Source: CAD feature listing. Evaluate the final solid. Frame: model axes, mm. Round coordinates to 2 decimals unless told otherwise and drop trailing zeros. Loops run counter-clockwise (first coordinate to the right, second up) from the corner with the lowest first, then second, coordinate; pieces in that order, holes last. Notation, with made-up numbers: M -13.75,12.25 L 11.25,12.25 A18 cw 11.25,25.25 Z; hole C -3,63 d3. An arc over 180 degrees is marked long. Write each question's results on one line, items separated by ' | '. Start each with the question number.
1. Section B-B on x = -120. Output: boundary loops of the cut face in (y, z) (1 decimal).
2. Section A-A on y = 117. Output: boundary loops of the cut face in (x, z) (1 decimal), and give its area (3 significant figures).
3. Section C-C on z = 2.2. Give the number of separate pieces and of enclosed holes in the cut face, and give its area (3 significant figures).
4. Ray query, line 1 (Y direction, x = 174.5, z = 0.6); line 2 (X direction, y = -81, z = 1.85); line 3 (X direction, y = -25.5, z = 2.6). Return the intervals inside material, ascending.
5. Contact query for flat-ended pins moving along their axis: pin 1 Ø5 at (x, y) = (-304.48, 86.35) entering from -Z; pin 2 Ø1 at (y, z) = (-46, 2) entering from +X; pin 3 Ø1.6 at (x, z) = (-8, 1) entering from +Y; pin 4 Ø1 at (y, z) = (166.5, 1) entering from -X. Output: stop coordinate, or through.
from build123d import *

# Parameters (mm, degrees)
SKETCH1_W                 = 570.860988324
SKETCH1_H                 = 315.575
BOSS_EXTRUDE1_DEPTH       = 3.175
SKETCH2_W                 = 3.175
SKETCH2_H                 = 101.6
CUT_EXTRUDE1_DEPTH        = 3.175
SKETCH7_W                 = 50
SKETCH7_H                 = 3.175
CUT_EXTRUDE5_DEPTH        = 3.175
LPATTERN2_COUNT           = 5
LPATTERN2_PITCH           = 91.96
LPATTERN2_COPY_1_SKETCH_W = 3.175
LPATTERN2_COPY_1_SKETCH_H = 101.6
LPATTERN2_COPY_1_DEPTH    = 3.175
LPATTERN2_COPY_2_SKETCH_W = 3.175
LPATTERN2_COPY_2_SKETCH_H = 101.6
LPATTERN2_COPY_2_DEPTH    = 3.175
LPATTERN2_COPY_3_SKETCH_W = 3.175
LPATTERN2_COPY_3_SKETCH_H = 101.6
LPATTERN2_COPY_3_DEPTH    = 3.175
LPATTERN2_COPY_4_SKETCH_W = 3.175
LPATTERN2_COPY_4_SKETCH_H = 101.6
LPATTERN2_COPY_4_DEPTH    = 3.175
SKETCH9_W                 = 95.12808
SKETCH9_H                 = 34.036
SKETCH9_R                 = 3.048
SKETCH9_W_2               = 34.036
SKETCH9_H_2               = 95.25
BOSS_EXTRUDE3_DEPTH       = 3.175
SKETCH10_W                = 3.175
SKETCH10_H                = 112.375
CUT_EXTRUDE6_DEPTH        = 373.646181611


with BuildPart() as part:
    # Sketch1 → Boss-Extrude1 (new body)
    with BuildSketch(Plane.XY):
        Rectangle(SKETCH1_W, SKETCH1_H)
    extrude(amount=BOSS_EXTRUDE1_DEPTH)

    # Sketch2 → Cut-Extrude1 (cut)
    with BuildSketch(Plane.XY.offset(3.175)):
        with Locations((-191.887994162, -81.5875)):
            Rectangle(SKETCH2_W, SKETCH2_H)
    cut_extrude1 = extrude(amount=-CUT_EXTRUDE1_DEPTH, mode=Mode.SUBTRACT)

    # Sketch7 → Cut-Extrude5 (cut)
    with BuildSketch(Plane.XY.offset(3.175)):
        with Locations((127.304934912, -156.2)):
            Rectangle(SKETCH7_W, SKETCH7_H)
        with Locations((-55.695065088, -156.2)):
            Rectangle(SKETCH7_W, SKETCH7_H)
    cut_extrude5 = extrude(amount=-CUT_EXTRUDE5_DEPTH, mode=Mode.SUBTRACT)

    # Mirror3: Cut-Extrude1 across plane
    add(cut_extrude1.mirror(Plane.ZX), mode=Mode.SUBTRACT)

    # LPattern2: Cut-Extrude1 ×5
    with Locations(*[(i * LPATTERN2_PITCH, 0, 0) for i in range(1, LPATTERN2_COUNT)]):
        add(cut_extrude1, mode=Mode.SUBTRACT)

    # LPattern2 copy 1 sketch → LPattern2 copy 1 (cut)
    with BuildSketch(Plane(origin=(91.96, 0, 3.175), x_dir=(1, 0, 0), z_dir=(0, 0, 1))):
        with Locations((-191.887994162, 81.5875)):
            Rectangle(LPATTERN2_COPY_1_SKETCH_W, LPATTERN2_COPY_1_SKETCH_H)
    extrude(amount=-LPATTERN2_COPY_1_DEPTH, mode=Mode.SUBTRACT)

    # LPattern2 copy 2 sketch → LPattern2 copy 2 (cut)
    with BuildSketch(Plane(origin=(183.92, 0, 3.175), x_dir=(1, 0, 0), z_dir=(0, 0, 1))):
        with Locations((-191.887994162, 81.5875)):
            Rectangle(LPATTERN2_COPY_2_SKETCH_W, LPATTERN2_COPY_2_SKETCH_H)
    extrude(amount=-LPATTERN2_COPY_2_DEPTH, mode=Mode.SUBTRACT)

    # LPattern2 copy 3 sketch → LPattern2 copy 3 (cut)
    with BuildSketch(Plane(origin=(275.88, 0, 3.175), x_dir=(1, 0, 0), z_dir=(0, 0, 1))):
        with Locations((-191.887994162, 81.5875)):
            Rectangle(LPATTERN2_COPY_3_SKETCH_W, LPATTERN2_COPY_3_SKETCH_H)
    extrude(amount=-LPATTERN2_COPY_3_DEPTH, mode=Mode.SUBTRACT)

    # LPattern2 copy 4 sketch → LPattern2 copy 4 (cut)
    with BuildSketch(Plane(origin=(367.84, 0, 3.175), x_dir=(1, 0, 0), z_dir=(0, 0, 1))):
        with Locations((-191.887994162, 81.5875)):
            Rectangle(LPATTERN2_COPY_4_SKETCH_W, LPATTERN2_COPY_4_SKETCH_H)
    extrude(amount=-LPATTERN2_COPY_4_DEPTH, mode=Mode.SUBTRACT)

    # Sketch9 → Boss-Extrude3 (add)
    # profile 1 of 3: a face of its own
    with BuildSketch(Plane(origin=(0, 0, 0), x_dir=(-1, 0, 0), z_dir=(0, 0, -1))):
        with Locations((-237.866454162, 174.8055)):
            Rectangle(SKETCH9_W, SKETCH9_H)
        with Locations((-260.030494162, 176.8375)):
            Circle(SKETCH9_R, mode=Mode.SUBTRACT)
    # profile 2 of 3: a face of its own
    with BuildSketch(Plane(origin=(0, 0, 0), x_dir=(-1, 0, 0), z_dir=(0, 0, -1))):
        with Locations((-302.448494162, 110.1625)):
            Rectangle(SKETCH9_W_2, SKETCH9_H_2)
        with Locations((-304.480494162, 86.35)):
            Circle(SKETCH9_R, mode=Mode.SUBTRACT)
        with Locations((-304.480494162, 133.975)):
            Circle(SKETCH9_R, mode=Mode.SUBTRACT)
    # profile 3 of 3: a face of its own
    with BuildSketch(Plane(origin=(0, 0, 0), x_dir=(-1, 0, 0), z_dir=(0, 0, -1))):
        with Locations((-302.448494162, -110.1625)):
            Rectangle(SKETCH9_W_2, SKETCH9_H_2)
        with Locations((-304.480494162, -133.975)):
            Circle(SKETCH9_R, mode=Mode.SUBTRACT)
        with Locations((-304.480494162, -86.35)):
            Circle(SKETCH9_R, mode=Mode.SUBTRACT)
    boss_extrude3 = extrude(amount=-BOSS_EXTRUDE3_DEPTH)

    # Mirror4: Boss-Extrude3 across plane
    add(boss_extrude3.mirror(Plane(origin=(0, 0, 0), x_dir=(0, 0, 1), z_dir=(1, 0, 0))))

    # Mirror5: Cut-Extrude5 across plane
    add(cut_extrude5.mirror(Plane.ZX), mode=Mode.SUBTRACT)

    # Sketch10 → Cut-Extrude6 (cut, through all)
    with BuildSketch(Plane(origin=(0, 0, 0), x_dir=(-1, 0, 0), z_dir=(0, 0, -1))):
        with Locations((-283.842994162, 0)):
            Rectangle(SKETCH10_W, SKETCH10_H)
    cut_extrude6 = extrude(amount=-CUT_EXTRUDE6_DEPTH, mode=Mode.SUBTRACT)

    # Mirror6: Cut-Extrude6 across plane
    add(cut_extrude6.mirror(Plane(origin=(0, 0, 0), x_dir=(0, 0, 1), z_dir=(1, 0, 0))), mode=Mode.SUBTRACT)


solid = part.part
Taken from the geometry:
1) outline: M -157.8,0 L 157.8,0 L 157.8,3.2 L -157.8,3.2 Z
2) outline: M -319.5,0 L -193.5,0 L -193.5,3.2 L -319.5,3.2 Z; M -190.3,0 L -101.5,0 L -101.5,3.2 L -190.3,3.2 Z; M -98.3,0 L -9.6,0 L -9.6,3.2 L -98.3,3.2 Z; M -6.4,0 L 82.4,0 L 82.4,3.2 L -6.4,3.2 Z; M 85.6,0 L 174.4,0 L 174.4,3.2 L 85.6,3.2 Z; M 177.5,0 L 319.5,0 L 319.5,3.2 L 177.5,3.2 Z | area: 1,980 mm^2
3) separate pieces: 1 | enclosed holes: 20 | area: 195,000 mm^2
4) line 1: -157.79 to -132.39, -30.79 to 30.79, 132.39 to 157.79 | line 2: -319.47 to -193.48, -190.3 to -101.52, -98.34 to -9.56, -6.38 to 82.4, 85.58 to 174.36, 177.54 to 319.47 | line 3: -282.26 to 282.26
5) pin 1: through | pin 2: x = 282.26 | pin 3: y = 157.79 | pin 4: x = -285.43
